Geometry check sheet. Reference: the model listing, model coordinates, mm. Coordinates: 2 decimals unless noted, no trailing zeros.
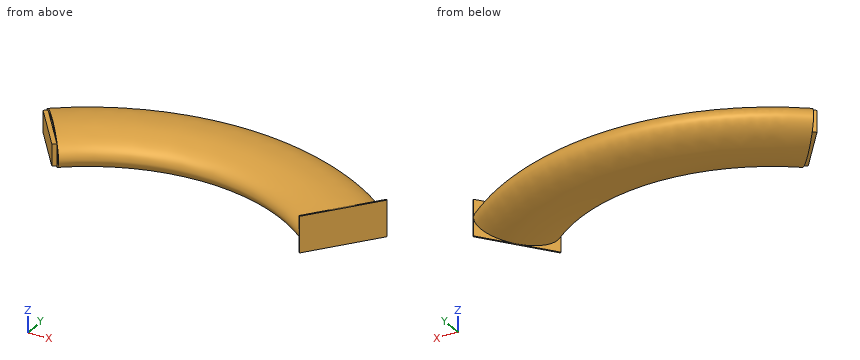
Autodesk Inventor part; units mm, degrees
ref_plane "Work Plane1" through (100, 0, 0) normal (-0.7817, 0.6236, 0) x (-0.6236, -0.7817, 0)
ref_plane "Work Plane2" through (-100, 0, 0) normal (-0.7817, -0.6236, 0) x (0, 0, 1)
ref_plane "YZ Plane" through (0, 0, 0) normal (1, 0, 0) x (0, 1, 0)
sketch "Sketch3" plane through (0, 0, 0) normal (0, 0, 1) x (1, 0, 0)
  line L0 (-140, 0) -> (140, 0)
  line L1 (0, -157.4286) -> (0, 67.0714)
  arc A0 (100, 0) -> (-100, 0) centre (0, -125.3571) ccw
  line L2 (-90.9685, 35) -> (88.04, 35) construction
  point P0 (0, 0)
  point P1 (0, 35)
  dimension "d0" = 200
  dimension "d1" = 35
ref_plane "Work Plane1" through (100, 0, 0) normal (-0.7817, 0.6236, 0) x (-0.6236, -0.7817, 0)
sketch "Sketch5" plane through (100, 0, 0) normal (-0.7817, 0.6236, 0) x (-0.6236, -0.7817, 0)
  ellipse E0 centre (0, 0) end of major axis (0, -12.5) minor radius 27.5
  ellipse E1 centre (0, 0) end of major axis (0, -10.5) minor radius 25.5
  point P0 (62.3608, 0)
  dimension "d2" = 27.5
  dimension "d3" = 12.5
  dimension "d4" = 25.5
  dimension "d5" = 10.5
sweep "Sweep1" add profiles "Sketch5" path "Sketch3" path curves A0
sketch "Sketch6" plane through (100, 0, 0) normal (-0.7817, 0.6236, 0) x (-0.6236, -0.7817, 0)
  line L0 (27.5, 12.5) -> (-27.5, 12.5)
  line L1 (-27.5, 12.5) -> (-27.5, -12.5)
  line L2 (-27.5, -12.5) -> (27.5, -12.5)
  line L3 (27.5, -12.5) -> (27.5, 12.5)
  line L4 (27.5, 12.5) -> (-27.5, -12.5) construction
  line L5 (-27.5, 12.5) -> (27.5, -12.5) construction
  point P0 (62.3608, 0)
  point P1 (0, 0)
  dimension "d8" = 55
  dimension "d9" = 25
extrude "Extrusion1" add sketch "Sketch6" against normal blind 1
ref_plane "Work Plane2" through (-100, 0, 0) normal (-0.7817, -0.6236, 0) x (0, 0, 1)
sketch "Sketch7" plane through (-100, 0, 0) normal (-0.7817, -0.6236, 0) x (0, 0, 1)
  line L0 (-7.5, -20) -> (7.5, -20)
  line L1 (7.5, -20) -> (7.5, 20)
  line L2 (7.5, 20) -> (-7.5, 20)
  line L3 (-7.5, 20) -> (-7.5, -20)
  line L4 (-7.5, -20) -> (7.5, 20) construction
  line L5 (7.5, -20) -> (-7.5, 20) construction
  point P0 (0, -62.3608)
  point P1 (0, 0)
  dimension "d12" = 15
  dimension "d13" = 40
extrude "Extrusion2" add sketch "Sketch7" along normal blind 3
equation "\"BendRadius\" = Thickness"
equation "\"BendReliefWidth\" = Thickness"
equation "\"BendReliefDepth\" = 0.5 * Thickness"
equation "\"CornerReliefSize\" = 4 * Thickness"
equation "\"MinimumRemnant\" = 2 * Thickness"
equation "\"TransitionRadius\" = BendRadius"
equation "\"JacobiRadiusSize\" = BendRadius"
equation "\"GapSize\" = Thickness"
properties part number "Handle bars holder"
1) Section check A-A on y = -7.5. Count the separate pieces of the cut face and the enclosed holes in it, and give its area (3 significant figures).
Data:
separate pieces: 3
enclosed holes: 1
area: 390 mm2
2) Material ranges on probe 1 along X at (y, z) = (-15, 2.25); probe 2 along Z at (x, y) = (-5.5, 57); probe 3 along X at (y, z) = (25, -4), recorded low to high.
Data:
probe 1: x = -91.87 to -88.03, -78.54 to -74.78, 74.78 to 78.54, 88.03 to 89.31
probe 2: z = -7.45 to -5.25, 5.25 to 7.45
probe 3: x = -110.19 to -105.95, 105.95 to 110.19
3) Depth check by flat-ended pin: pin 1 (12 mm diameter, centred on x = 31, y = 6, fed in from +Z); pin 2 (12 mm diameter, centred on x = 49.5, z = 10, fed in from +Y); pin 3 (6 mm diameter, centred on x = -87.5, z = -6, fed in from -Y). Enter the tip coordinate at first touch or a pass-through.
Data:
pin 1: stops at z = 8.86
pin 2: stops at y = 54.63
pin 3: stops at y = -19.36
